Verification items for the finished model (mm, model axes). Coordinates: 2 decimals unless noted, no trailing zeros. Order: outer loops, then holes, each group sorted by start corner. A loop starts at its lowest first (then second) coordinate and runs counter-clockwise, first axis right, second up. Notation, with made-up numbers: M 86,31 L 111,31 A24 ccw 111,62 Z; hole C 27,42 d5. An arc over 180 degrees is marked long. Write item = value, one per line.
```python
from build123d import *

# Parameters (mm, degrees)
SKETCH1_R           = 4
SKETCH1_R_2         = 0.7
BOSS_EXTRUDE1_DEPTH = 4


with BuildPart() as part:
    # Sketch1 → Boss-Extrude1 (new body)
    with BuildSketch(Plane(origin=(0, 0, 0), x_dir=(0, 0, -1), z_dir=(1, 0, 0))):
        with BuildLine():
            Line((-70, 15.254804339), (-70, -15.254804339))
            Line((-70, -15.254804339), (0.489836976, -12.490398702))
            ThreePointArc((0.489836976, -12.490398702), (12.5, 0), (0.489836976, 12.490398702))
            Line((0.489836976, 12.490398702), (-70, 15.254804339))
        make_face()
        Circle(SKETCH1_R, mode=Mode.SUBTRACT)
        with Locations((-7.24, 0)):
            Circle(SKETCH1_R_2, mode=Mode.SUBTRACT)
        with Locations((0, 7.24)):
            Circle(SKETCH1_R_2, mode=Mode.SUBTRACT)
        with Locations((7.24, 0)):
            Circle(SKETCH1_R_2, mode=Mode.SUBTRACT)
        with Locations((0, -7.24)):
            Circle(SKETCH1_R_2, mode=Mode.SUBTRACT)
    extrude(amount=BOSS_EXTRUDE1_DEPTH)


solid = part.part
```
Item 1: Sectioned sample at B-B, the plane y = -9. Enter the section's corners in (x, z).
Report:
outline = M 0,-8.67 L 4,-8.67 L 4,70 L 0,70 Z
Item 2: Scan lines: L1, parallel to Y at x = 3.25, z = -1; L2, parallel to Y at x = 3.1, z = 0; L3, parallel to Y at x = 3.65, z = 2.5. Record each from-to range of solid material in increasing order. Write a range as from..to.
Report:
L1 = -12.46..-3.87, 3.87..12.46
L2 = -12.51..-7.94, -6.54..-4, 4..6.54, 7.94..12.51
L3 = -12.61..-3.12, 3.12..12.61
Item 3: Sectioned sample at A-A, the plane x = 3.05. Enter the section's corners in (y, z).
Report:
outline = M -15.25,70 L -12.49,-0.49 A12.5 ccw 12.49,-0.49 L 15.25,70 Z; hole C -7.24,0 d1.4; hole C 0,0 d8; hole C 0,-7.24 d1.4; hole C 0,7.24 d1.4; hole C 7.24,0 d1.4
Item 4: Sectioned sample at C-C, the plane z = 30. Enter the section's corners in (x, y).
Report:
outline = M 0,-13.69 L 4,-13.69 L 4,13.69 L 0,13.69 Z
Item 5: Gauge pin test, flat ends, axial feed: pin 1 (1.5 mm diameter, centred on y = -10, z = 13.5, fed in from -X); pin 2 (1 mm diameter, centred on x = 1.5, z = -2.5, fed in from -Y); pin 3 (0.8 mm diameter, centred on y = -7.24, z = 0, fed in from +X). Record the tip position at first contact, or that the pin passes through.
Report:
pin_1 = 0
pin_2 = -12.34
pin_3 = through
Item 6: Release check for a two-part mould opening along Y. For faces 1 (the cylindrical face through (1.972, 6.557, 0.152)), 2 (the flat face through (1.972, -13.892, 35.249)), 3 (the flat face through (1.972, 13.853, 34.262)) record: pulls with the +Y half, pulls with the -Y half, needs draft (parallel to the pull), parting line crosses it, or undercut.
Report:
face_1 = undercut
face_2 = pulls with the -Y half
face_3 = pulls with the +Y half
